Read the model definition and answer for the solid it produces. Units are mm, in the model's axes. A direction names the side the tool comes from. Round coordinates to 2 decimals unless told otherwise and drop trailing zeros. Order: outer loops, then holes, each group sorted by start corner. A loop starts at its lowest first (then second) coordinate and runs counter-clockwise, first axis right, second up. Notation, with made-up numbers: M 11.25,-21 L 56.25,-21 A22 ccw 56.25,8 Z; hole C -13.75,66.5 d9. An arc over 180 degrees is marked long. Use one line per item in the form item = value. Start each with the question number.
from build123d import *

# Parameters (mm, degrees)
F0_W     = 660.4
F0_H     = 50.8
F1_DEPTH = 9.525
F2_W     = 12.7
F2_H     = 44.45
F3_W     = 12.7
F3_H     = 44.45
F4_DEPTH = 38.1
F5_DEPTH = 38.1


with BuildPart() as f1:
    # F0 (on Front) → F1 (new body, symmetric)
    with BuildSketch(Plane.XZ):
        Rectangle(F0_W, F0_H)
    extrude(amount=F1_DEPTH, both=True)

    # F2 (on face) + F3 (on face) → F4 (join)
    with BuildSketch(Plane(origin=(-330.2, 0, 0), x_dir=(0, -1, 0), z_dir=(-1, 0, 0))):
        Rectangle(F2_W, F2_H)
    with BuildSketch(Plane.YZ.offset(330.2)):
        Rectangle(F3_W, F3_H)
    extrude(amount=F4_DEPTH)

    # F3 (on face) → F5 (join)
    with BuildSketch(Plane.YZ.offset(330.2)):
        Rectangle(F3_W, F3_H)
    extrude(amount=F5_DEPTH)


solid = f1.part
Item 1: Given P1, Ø6.5, axis at x = -351.5, y = -0.5, coming from the -Z side (3 decimals), flat-ended and moving along its own axis, determine where the tip first touches the part or whether it passes through.
Item 2: Section A-A (z = -6.5) is taken. Write down the section's boundary in (x, y) (3 decimals).
Item 3: Find the intervals of material crossed by L1, parallel to X at y = 8, z = 9, in increasing order. Write a range as [from, to].
Item 4: A tool of negligible diameter and unlimited length cuts with its end or side. For faces 1 (the flat face through (349, 6.35, 0)), 2 (the flat face through (349, -6.35, 0)), 3 (the flat face through (349, 0, -22.225)), 4 (the flat face through (-349, 6.35, 0)), from which of +Z, -Z, +X, -X, +Y, -Y can it reach the whole face along a straight path? Write none if from no direction.
The answers:
q1.P1 = -22.225
q2.outline = M -368.3,-6.35 L -330.2,-6.35 L -330.2,-9.525 L 330.2,-9.525 L 330.2,-6.35 L 368.3,-6.35 L 368.3,6.35 L 330.2,6.35 L 330.2,9.525 L -330.2,9.525 L -330.2,6.35 L -368.3,6.35 Z
q3.L1 = [-330.2, 330.2]
q4.face_1 = +Z, -Z, +X, +Y
q4.face_2 = +Z, -Z, +X, -Y
q4.face_3 = -Z, +X, +Y, -Y
q4.face_4 = +Z, -Z, -X, +Y
